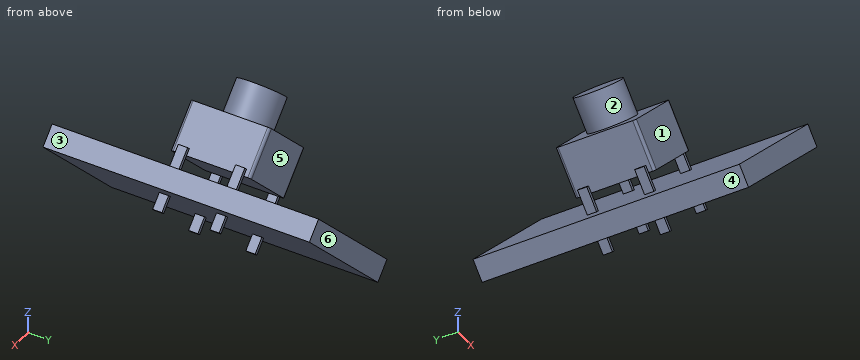
from build123d import *

# Parameters (mm, degrees)
BOX026_W              = 12
BOX026_H              = 20
BOX026_DEPTH          = 1.6
BOX026_PITCH_ANGLE    = -45
BOX024_W              = 0.3
BOX024_H              = 0.7
BOX024_DEPTH          = 4.5
BOX021_W              = 0.3
BOX021_H              = 0.7
BOX021_DEPTH          = 4.5
BOX025_W              = 0.3
BOX025_H              = 0.7
BOX025_DEPTH          = 4.5
BOX022_W              = 0.3
BOX022_H              = 0.7
BOX022_DEPTH          = 4.5
CYLINDER042_R         = 1.75
CYLINDER042_DEPTH     = 6
BOX023_W              = 6
BOX023_H              = 6
BOX023_DEPTH          = 3.5
FILLET004_R           = 0.2
FUSION004_PITCH_ANGLE = -45


with BuildPart() as obj1:
    # Box026 → Box026 (new body)
    with BuildSketch(Plane.XY):
        with Locations((6, 10)):
            Rectangle(BOX026_W, BOX026_H)
    extrude(amount=BOX026_DEPTH)


with BuildPart() as obj1_1:
    # Box026 pitch: moved
    add(obj1.part.rotate(Axis((0, 0, 0), (0, 1, 0)), BOX026_PITCH_ANGLE))


with BuildPart() as obj1_2:
    # Box026 placement: moved
    add(obj1_1.part.moved(Location((-43, -10, 4))))


with BuildPart() as cubo021:
    # Box024 → Box024 (new body)
    with BuildSketch(Plane(origin=(6, 0.5, -4), x_dir=(1, 0, 0), z_dir=(0, 0, 1))):
        with Locations((0.15, 0.35)):
            Rectangle(BOX024_W, BOX024_H)
    extrude(amount=BOX024_DEPTH)


with BuildPart() as cubo018:
    # Box021 → Box021 (new body)
    with BuildSketch(Plane(origin=(6, 4.8, -4), x_dir=(1, 0, 0), z_dir=(0, 0, 1))):
        with Locations((0.15, 0.35)):
            Rectangle(BOX021_W, BOX021_H)
    extrude(amount=BOX021_DEPTH)


with BuildPart() as cubo022:
    # Box025 → Box025 (new body)
    with BuildSketch(Plane(origin=(-0.3, 4.8, -4), x_dir=(1, 0, 0), z_dir=(0, 0, 1))):
        with Locations((0.15, 0.35)):
            Rectangle(BOX025_W, BOX025_H)
    extrude(amount=BOX025_DEPTH)


with BuildPart() as cubo019:
    # Box022 → Box022 (new body)
    with BuildSketch(Plane(origin=(-0.3, 0.5, -4), x_dir=(1, 0, 0), z_dir=(0, 0, 1))):
        with Locations((0.15, 0.35)):
            Rectangle(BOX022_W, BOX022_H)
    extrude(amount=BOX022_DEPTH)


with BuildPart() as cilindro018:
    # Cylinder042 → Cylinder042 (new body)
    with BuildSketch(Plane(origin=(3, 3, 0), x_dir=(1, 0, 0), z_dir=(0, 0, 1))):
        Circle(CYLINDER042_R)
    extrude(amount=CYLINDER042_DEPTH)


with BuildPart() as obj2:
    # Box023 → Box023 (new body)
    with BuildSketch(Plane.XY):
        with Locations((3, 3)):
            Rectangle(BOX023_W, BOX023_H)
    extrude(amount=BOX023_DEPTH)

    # Fillet004
    fillet004_edges = [obj2.edges().sort_by_distance(p)[0] for p in [
        (0, 0, 1.75),
        (0, 6, 1.75),
        (6, 0, 1.75),
        (6, 6, 1.75),
    ]]
    fillet(fillet004_edges, radius=FILLET004_R)

    # Fusion004: union Cubo021, Cubo018, Cubo022, Cubo019, Cilindro018
    add(cubo021.part)
    add(cubo018.part)
    add(cubo022.part)
    add(cubo019.part)
    add(cilindro018.part)


with BuildPart() as obj2_1:
    # Fusion004 pitch: moved
    add(obj2.part.rotate(Axis((0, 0, 0), (0, 1, 0)), FUSION004_PITCH_ANGLE))


with BuildPart() as obj2_2:
    # Fusion004 placement: moved
    add(obj2_1.part.moved(Location((-43, -3, 8))))

    # Fusion005: union obj1
    add(obj1_2.part)


with BuildPart() as obj2_3:
    # Fusion005 placement: moved
    add(obj2_2.part.moved(Location((1.5, 0, 0))))


solid = obj2_3.part
Can you work these out from the model? Positions are in its coordinate system, mm. Face numbers are marked on the shaded views. A direction names the side the tool comes from. Give positions to 0.01 mm unless a question says otherwise; leave off trailing zeros. Loops run counter-clockwise (first coordinate to the right, second up) from the corner with the lowest first, then second, coordinate; pieces in that order, holes last. Notation, with made-up numbers: (77, 4) -> (105, 4) arc R16 ccw to (105, 25) -> close; hole circle Ø5 at (74, -16.75). An arc over 180 degrees is marked (long way). Use one line per item in the form item = value.
1) If we section it at B-B (z = 5.5): Please give me the cut outline in (x, y), plus the area to 3 significant figures.
Answers:
outline = (-42.26, -10) -> (-40, -10) -> (-40, 10) -> (-42.26, 10) -> close; (-39.42, -2.5) -> (-39, -2.5) -> (-39, -1.8) -> (-39.42, -1.8) -> close; (-39.42, 1.8) -> (-39, 1.8) -> (-39, 2.5) -> (-39.42, 2.5) -> close
area = 45.8 mm²
2) If we section it at D-D (y = 6.75): Please give me the cut outline in (x, z), plus the area to 3 significant figures.
Answers:
outline = (-42.63, 5.13) -> (-41.5, 4) -> (-33.01, 12.49) -> (-34.15, 13.62) -> close
area = 19.2 mm²
3) If we section it at A-A (y = 1): Please give me the cut outline in (x, z).
Answers:
outline = (-44.64, 13.35) -> (-42.87, 11.58) -> (-43.97, 10.47) -> (-41.5, 8) -> (-37.26, 12.24) -> (-39.73, 14.72) -> (-40.84, 13.61) -> (-42.61, 15.38) -> close; (-42.63, 5.13) -> (-41.5, 4) -> (-33.01, 12.49) -> (-34.15, 13.62) -> close
4) If we section it at C-C (x = -34.75): Please give me the cut outline in (y, z).
Answers:
outline = (-10, 10.75) -> (10, 10.75) -> (10, 13.01) -> (-10, 13.01) -> close; (-2.5, 9.74) -> (-1.8, 9.74) -> (-1.8, 10.16) -> (-2.5, 10.16) -> close; (1.8, 9.74) -> (2.5, 9.74) -> (2.5, 10.16) -> (1.8, 10.16) -> close
5) I need wall thicknesses on line 1 along Y through (x, z) = (-40, 13.75); line 2 along X through (y, z) = (-2.25, 7.25); line 3 along X through (y, z) = (-0.25, 10.5). Which ranges of each line are inside material? Lowest first, please.
Answers:
line_1 = -3 to 3
line_2 = -41.17 to -40.75, -40.51 to -38.25
line_3 = -43.95 to -39, -37.26 to -35
6) Will these pins go through, and if not, where does the flat tip stop? pin 1 (2 mm diameter, centred on x = -36.5, y = 2, fed in from -Z); pin 2 (1.6 mm diameter, centred on x = -37, z = 12, fed in from +Y); pin 3 (1.1 mm diameter, centred on x = -39, z = 5.5, fed in from +Y); pin 4 (0.8 mm diameter, centred on x = -39.5, z = 5.5, fed in from -Y).
Answers:
pin_1 = 8
pin_2 = 3
pin_3 = 2.5
pin_4 = -10
7) For the marked faces 5 and 6, which set-ups out of +Z, -Z, +X, -X, +Y, -Y let a thin tool reach every point of the face, with its end or its side?
Answers:
face_5 = +Z, -X, +Y
face_6 = +Z, -Z, +X, -X, +Y
8) We'd pull the mould along X, two halves only. Please class the marked faces 1, 2, 3 and 4: released by +X, released by -X, zero draft, split by the parting line, or undercut.
Answers:
face_1 = zero draft
face_2 = undercut
face_3 = released by +X
face_4 = released by -X
